```python
from build123d import *

# Parameters (mm, degrees)
SKETCH1_W           = 1371.6
SKETCH1_H           = 88.9
BOSS_EXTRUDE1_DEPTH = 38.1
CUT_EXTRUDE1_REACH  = 40.1
CUT_EXTRUDE2_REACH  = 40.1
CUT_EXTRUDE3_DEPTH  = 9.525


with BuildPart() as part:
    # Sketch1 → Boss-Extrude1 (new body)
    with BuildSketch(Plane.XY):
        with Locations((685.8, 44.45)):
            Rectangle(SKETCH1_W, SKETCH1_H)
    extrude(amount=BOSS_EXTRUDE1_DEPTH)

    # Sketch2 → Cut-Extrude1 (cut, up to next)
    with BuildSketch(Plane.XY.offset(38.1), mode=Mode.PRIVATE) as cut_extrude1_sk1:
        Polygon((0, 88.9), (88.9, 0), (0, 0), align=None)
    cut_extrude1_tool1 = extrude(cut_extrude1_sk1.sketch, amount=-CUT_EXTRUDE1_REACH, mode=Mode.PRIVATE) & part.part
    add(cut_extrude1_tool1.solids().sort_by_distance((29.633333, 29.633333, 38.1))[0], mode=Mode.SUBTRACT)

    # Sketch3 → Cut-Extrude2 (cut, up to next)
    with BuildSketch(Plane.XY.offset(38.1), mode=Mode.PRIVATE) as cut_extrude2_sk1:
        Polygon((1371.6, 88.9), (1282.7, 0), (1371.6, 0), align=None)
    cut_extrude2_tool1 = extrude(cut_extrude2_sk1.sketch, amount=-CUT_EXTRUDE2_REACH, mode=Mode.PRIVATE) & part.part
    add(cut_extrude2_tool1.solids().sort_by_distance((1341.966667, 29.633333, 38.1))[0], mode=Mode.SUBTRACT)

    # Sketch4 → Cut-Extrude3 (cut)
    with BuildSketch(Plane.XY.offset(38.1)):
        Polygon((88.9, 0), (1282.7, 0), (1295.4, 12.7), (76.2, 12.7), align=None)
    extrude(amount=-CUT_EXTRUDE3_DEPTH, mode=Mode.SUBTRACT)


solid = part.part
```
Check sheet for the modelled part. Datum: model origin and axes. Units: mm. Round coordinates to 2 decimals unless told otherwise and drop trailing zeros. Write each loop counter-clockwise with the first axis right and the second up, starting at its lowest first coordinate (ties: lowest second). Pieces come first, ordered by that corner, then holes. Notation, with made-up numbers: (36, -28.5) -> (80, -28.5) arc R20 ccw to (80, -16.5) -> close; hole circle Ø7 at (81.5, -29.75). An arc over 180 degrees is marked (long way). One line per question, with ' | ' between items. Start each with the question number.
1. Sectioned sample at B-B, the plane y = 35.5. Record the cut outline in (x, z), then the cut area to 3 significant figures.
2. Sectioned sample at A-A, the plane x = 362.5. Record the cut outline in (y, z) (3 decimals), then the cut area to 3 significant figures.
3. Scan lines: line 1 along Y through (x, z) = (897.5, 30); line 2 along Z through (x, y) = (142, 4.5) (3 decimals); line 3 along X through (y, z) = (25, 7). Record each from-to range of solid material in increasing order. Write a range as from..to.
4. Depth check by flat-ended pin: pin 1 (1 mm diameter, centred on x = 1000, y = 56, fed in from -Z); pin 2 (7.5 mm diameter, centred on x = 525, z = 33, fed in from -Y); pin 3 (4 mm diameter, centred on x = 477.5, y = 8, fed in from +Z) (3 decimals); pin 4 (12 mm diameter, centred on y = 58.5, z = 16, fed in from +X). Enter the tip coordinate at first touch or a pass-through.
5. Sectioned sample at C-C, the plane z = 19. Record the cut outline in (x, y).
Taken from the geometry:
1) outline: (53.4, 0) -> (1318.2, 0) -> (1318.2, 38.1) -> (53.4, 38.1) -> close | area: 48,200 mm^2
2) outline: (0, 0) -> (88.9, 0) -> (88.9, 38.1) -> (12.7, 38.1) -> (12.7, 28.575) -> (0, 28.575) -> close | area: 3,270 mm^2
3) line 1: y = 12.7..88.9 | line 2: z = 0..28.575 | line 3: x = 63.9..1307.7
4) pin 1: stops at z = 0 | pin 2: stops at y = 12.7 | pin 3: stops at z = 28.575 | pin 4: stops at x = 1347.2
5) outline: (0, 88.9) -> (88.9, 0) -> (1282.7, 0) -> (1371.6, 88.9) -> close
